```python
from build123d import *

# Parameters (mm, degrees)
SKETCH_1_R          = 2.5
EXTRUDE_1_DEPTH     = 4
EXTRUDE_2_DEPTH     = 20.7
SKETCH_3_R          = 3
CUT_EXTRUDE_1_DEPTH = 6.7
CUT_EXTRUDE_2_DEPTH = 10


with BuildPart() as part:
    # Эскиз1 → Бобышка-Вытянуть1 (new body)
    with BuildSketch(Plane.XY):
        Polygon((0, 0), (108, 0), (108, 30), (55, 50), (55, 68), (0, 68), align=None)
        with Locations((21, 57)):
            Circle(SKETCH_1_R, mode=Mode.SUBTRACT)
        with Locations((49, 57)):
            Circle(SKETCH_1_R, mode=Mode.SUBTRACT)
        with Locations((21, 11)):
            Circle(SKETCH_1_R, mode=Mode.SUBTRACT)
        with Locations((49, 11)):
            Circle(SKETCH_1_R, mode=Mode.SUBTRACT)
        with Locations((88, 15)):
            Circle(SKETCH_1_R, mode=Mode.SUBTRACT)
    extrude(amount=EXTRUDE_1_DEPTH)

    # Эскиз2 → Бобышка-Вытянуть2 (add)
    with BuildSketch(Plane.XY.offset(4)):
        Polygon((108, 0), (104, 0), (104, 31.509433962), (108, 30), align=None)
    extrude(amount=-EXTRUDE_2_DEPTH)

    # Эскиз3 → Вырез-Вытянуть1 (cut)
    with BuildSketch(Plane(origin=(108, 0, 0), x_dir=(0, 0, -1), z_dir=(1, 0, 0))):
        with Locations((6, 10)):
            Circle(SKETCH_3_R)
    extrude(amount=-CUT_EXTRUDE_1_DEPTH, mode=Mode.SUBTRACT)

    # Эскиз4 → Вырез-Вытянуть2 (cut)
    with BuildSketch(Plane(origin=(0, 0, 0), x_dir=(-1, 0, 0), z_dir=(0, 0, -1))):
        Polygon((0, 68), (-15, 68), (-15, 48), (-15, 28), (-10, 28), (-10, 58), (0, 58), align=None)
    extrude(amount=-CUT_EXTRUDE_2_DEPTH, mode=Mode.SUBTRACT)


solid = part.part
```
Work out the finished part from the listing and answer in its coordinate system (mm). A direction names the side the tool comes from. Give positions to 0.01 mm unless a question says otherwise; leave off trailing zeros. Order: outer loops, then holes, each group sorted by start corner. A loop starts at its lowest first (then second) coordinate and runs counter-clockwise, first axis right, second up. Notation, with made-up numbers: (-38, 43.25) - (3, 43.25) arc R36 ccw to (3, 82.25) - close; hole circle Ø7 at (32, 24). An arc over 180 degrees is marked (long way). One line per item, written item: value. Start each with the question number.
1. Section C-C, the plane z = 2.25 is taken. Write down the section's boundary in (x, y).
2. Section A-A, the plane y = 15 is taken. Write down the section's boundary in (x, z), then the cut area to 3 significant figures.
3. Section B-B, the plane x = 21 is taken. Write down the section's boundary in (y, z), then the cut area to 3 significant figures.
4. Which of the six approach directions +Z, -Z, +X, -X, +Y, -Y give full straight-line access (tool end or side, diameter ignored) to faces 5 (the face through (5, 58, 2)), 6 (the face through (18.5, 57.1, 2)), 7 (the face through (13, 28, 2)), 8 (the face through (104, 16, -8))?
5. Section D-D, the plane z = -14.5 is taken. Write down the section's boundary in (x, y).
6. Each of these flat-tipped pins is pushed along its axis until it touches: pin 1 Ø1.2 at (y, z) = (46, 3) entering from -X; pin 2 Ø6 at (y, z) = (13, -5) entering from -X; pin 3 Ø3 at (x, y) = (43.5, 11.5) entering from -Z; pin 4 Ø3 at (x, z) = (5, 2) entering from +Y. Where does it stop, or does it pass through?
7. Consider line 1 (Y direction, x = 21, z = 3.2); line 2 (X direction, y = 53.5, z = 2.25); line 3 (Z direction, x = 80, y = 17). Determine where each line is inside the solid, lowest interval first.
8. For a pull along X with two mould halves and no side action, classify faces 1 (the face through (0, 29, 2)), 2 (the face through (51.31, 56.04, 1.97)), 3 (the face through (41, 27, 4)), 4 (the face through (108, 15, -6)) as released by +X, released by -X, zero draft, split by the parting line, or undercut.
Filled sheet:
1. outline: (0, 0) - (108, 0) - (108, 30) - (55, 50) - (55, 68) - (15, 68) - (15, 28) - (10, 28) - (10, 58) - (0, 58) - close; hole circle Ø5 at (21, 11); hole circle Ø5 at (21, 57); hole circle Ø5 at (49, 11); hole circle Ø5 at (49, 57); hole circle Ø5 at (88, 15)
2. outline: (0, 0) - (85.5, 0) - (85.5, 4) - (0, 4) - close; (90.5, 0) - (104, 0) - (104, -16.7) - (108, -16.7) - (108, 4) - (90.5, 4) - close
2. area: 479 mm²
3. outline: (0, 0) - (8.5, 0) - (8.5, 4) - (0, 4) - close; (13.5, 0) - (54.5, 0) - (54.5, 4) - (13.5, 4) - close; (59.5, 0) - (68, 0) - (68, 4) - (59.5, 4) - close
3. area: 232 mm²
4. face 5: +Z, -Z, -X, +Y
4. face 6: +Z, -Z
4. face 7: +Z, -Z, +Y
4. face 8: -Z, -X, +Y, -Y
5. outline: (104, 0) - (108, 0) - (108, 30) - (104, 31.51) - close
6. pin 1: x = 0
6. pin 2: x = 104
6. pin 3: z = 0
6. pin 4: y = 58
7. line 1: 0 to 8.5, 13.5 to 54.5, 59.5 to 68
7. line 2: 0 to 10, 15 to 55
7. line 3: 0 to 4
8. face 1: released by -X
8. face 2: undercut
8. face 3: zero draft
8. face 4: released by +X
